from build123d import *

# Parameters (mm, degrees)
SKETCH1_R           = 10.25
BOSS_EXTRUDE1_DEPTH = 15
SKETCH2_R           = 7.5
CUT_EXTRUDE1_DEPTH  = 15
FILLET1_R           = 0.5


with BuildPart() as part:
    # Sketch1 → Boss-Extrude1 (new body)
    with BuildSketch(Plane(origin=(0, 0, 0), x_dir=(1, 0, 0), z_dir=(0, 1, 0))):
        with Locations(Location((0, 0, 0), (0, 0, 270))):
            Circle(SKETCH1_R)
    extrude(amount=BOSS_EXTRUDE1_DEPTH)

    # Sketch2 → Cut-Extrude1 (cut)
    with BuildSketch(Plane(origin=(0, 15, 0), x_dir=(1, 0, 0), z_dir=(0, 1, 0))):
        with Locations(Location((0, 0, 0), (0, 0, 270))):
            Circle(SKETCH2_R)
    extrude(amount=-CUT_EXTRUDE1_DEPTH, mode=Mode.SUBTRACT)

    # Fillet1
    fillet1_edges = [part.edges().sort_by_distance(p)[0] for p in [
        (0, 0, -10.25),
    ]]
    fillet(fillet1_edges, radius=FILLET1_R)


solid = part.part
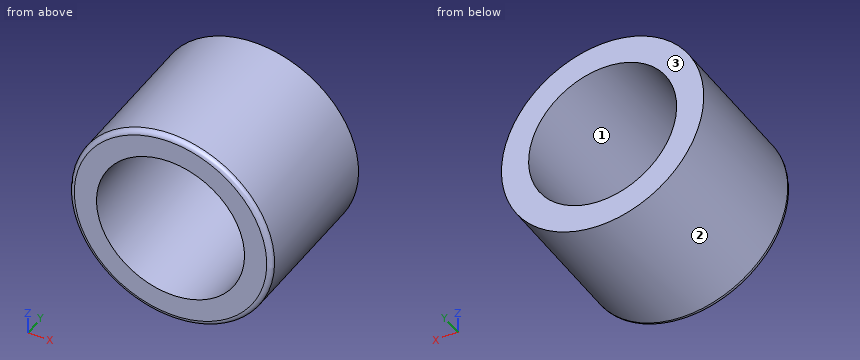
Part model, mm, in its own coordinate system. Face numbers are marked on the shaded views. Coordinates: 2 decimals unless noted, no trailing zeros. Loops run counter-clockwise (first coordinate to the right, second up) from the corner with the lowest first, then second, coordinate; pieces in that order, holes last. Notation, with made-up numbers: (-1, -30) -> (30, -30) arc R17 cw to (30, -1) -> close; hole circle Ø8 at (-16.5, 38). An arc over 180 degrees is marked (long way). Use a Markdown table: item, result. Add a question column.
Item 1: Pull direction Z, two halves, no side cores. Call the marked faces 1, 2 and 3: +Z half, -Z half, draft (parallel to the pull), parting line (faces both ways), or undercut.
Item 2: Band-saw the part on B-B on z = 0. Write the cut outline in (x, y).
Item 3: Flat gauge pins, fed straight in: P1, Ø3, axis at x = -4.5, y = 4.5, coming from the +Z side; P2, Ø3, axis at x = 7.5, z = 8, coming from the +Y side; P3, Ø3, axis at y = 4.5, z = 7, coming from the +X side; P4, Ø5, axis at x = 3, y = 8.5, coming from the +Z side. Where does each tip first touch, or does it go through?
Item 4: Band-saw the part on A-A on x = 0. Write the cut outline in (y, z), plus the area to 3 significant figures.
Item 5: Probe probe 1 along X at (y, z) = (7.5, 0); probe 2 along Z at (x, y) = (-0.75, 1.5); probe 3 along Z at (x, y) = (1.75, 4.25). List the from-to ranges inside material, lowest first.
Item 6: Band-saw the part on C-C on y = 7.25. Write the cut outline in (x, z).
Geometry says:
| question | item | result |
|---|---|---|
| 1 | face 1 | undercut |
| 1 | face 2 | parting line |
| 1 | face 3 | draft |
| 2 | outline | (-10.25, 0.5) arc R0.5 ccw to (-9.75, 0) -> (-7.5, 0) -> (-7.5, 15) -> (-10.25, 15) -> close; (7.5, 0) -> (9.75, 0) arc R0.5 ccw to (10.25, 0.5) -> (10.25, 15) -> (7.5, 15) -> close |
| 3 | P1 | z = 9.8 |
| 3 | P2 | y = 15 |
| 3 | P3 | x = 8.65 |
| 3 | P4 | z = 10.24 |
| 4 | outline | (0, -9.75) arc R0.5 ccw to (0.5, -10.25) -> (15, -10.25) -> (15, -7.5) -> (0, -7.5) -> close; (0, 7.5) -> (15, 7.5) -> (15, 10.25) -> (0.5, 10.25) arc R0.5 ccw to (0, 9.75) -> close |
| 4 | area | 82.4 mm² |
| 5 | probe 1 | -10.25 to -7.5, 7.5 to 10.25 |
| 5 | probe 2 | -10.22 to -7.46, 7.46 to 10.22 |
| 5 | probe 3 | -10.1 to -7.29, 7.29 to 10.1 |
| 6 | outline | circle Ø20.5 at (0, 0); hole circle Ø15 at (0, 0) |
